```python
from build123d import *

# Parameters (mm, degrees)
F0_W     = 160
F0_H     = 97
F1_DEPTH = 42
F2_R     = 1.725
F3_DEPTH = 3
F4_R     = 1.725
F5_DEPTH = 3


with BuildPart() as f1:
    # F0 (on Top) → F1 (new body)
    with BuildSketch(Plane.XY):
        with Locations((80, 48.5)):
            Rectangle(F0_W, F0_H)
    extrude(amount=F1_DEPTH)

    # F2 (on face) → F3 (cut)
    with BuildSketch(Plane.XZ):
        with Locations((140, 10)):
            Circle(F2_R)
        with Locations((140, 28)):
            Circle(F2_R)
        with Locations((22, 19.5)):
            Circle(F2_R)
    extrude(amount=-F3_DEPTH, mode=Mode.SUBTRACT)

    # F4 (on face) → F5 (cut)
    with BuildSketch(Plane(origin=(0, 0, 0), x_dir=(1, 0, 0), z_dir=(0, 0, -1))):
        with Locations((4.8, -91.8)):
            Circle(F4_R)
        with Locations((24, -32.5)):
            Circle(F4_R)
        with Locations((148.5, -91.8)):
            Circle(F4_R)
        with Locations((102, -32.5)):
            Circle(F4_R)
    extrude(amount=-F5_DEPTH, mode=Mode.SUBTRACT)


solid = f1.part
```
Work out the finished part from the listing and answer in its coordinate system (mm). A direction names the side the tool comes from. Round coordinates to 2 decimals unless told otherwise and drop trailing zeros. Return JSON: item names as keys, results as strings. Group by question number.
Q1. For faces 1 (the flat face through (79, 49, 0)), 2 (the cylindrical face through (21.626, 1.479, 17.816)), 3 (the cylindrical face through (103.593, 33.161, 1.479)), determine the directions among +Z, -Z, +X, -X, +Y, -Y from which every point of the face is accessible in a straight line to the end or side of a thin tool.
Q2. The mould has two halves that part along Y. Classify faces 4 (the cylindrical face through (4.426, 93.484, 1.479)), 5 (the flat face through (140, 3, 10)), 6 (the flat face through (0, 48, 21)): released by +Y, released by -Y, zero draft, split by the parting line, or undercut.
Q3. Find the intervals of material crossed by L1, parallel to X at y = 91.8, z = 0.95 (3 decimals); L2, parallel to Z at x = 140, y = 1 (3 decimals); L3, parallel to Y at x = 24, z = 2.1 (3 decimals), in increasing order.
Q4. Each of these flat-tipped pins is pushed along its axis until it touches: pin 1 Ø1 at (x, z) = (140, 10) entering from -Y; pin 2 Ø1.7 at (x, y) = (24, 32) entering from -Z. Where does it stop, or does it pass through?
Solved:
{
 "1": {"face 1": "-Z, +X, -X, +Y, -Y", "face 2": "-Y", "face 3": "-Z"},
 "2": {"face 4": "undercut", "face 5": "released by -Y", "face 6": "zero draft"},
 "3": {"L1": "0 to 3.075, 6.525 to 146.775, 150.225 to 160", "L2": "0 to 8.275, 11.725 to 26.275, 29.725 to 42", "L3": "0 to 30.775, 34.225 to 97"},
 "4": {"pin 1": "y = 3", "pin 2": "z = 3"}
}
